Read the model definition and answer for the solid it produces. Units are mm, in the model's axes. A direction names the side the tool comes from. Round coordinates to 2 decimals unless told otherwise and drop trailing zeros. Loops run counter-clockwise (first coordinate to the right, second up) from the corner with the lowest first, then second, coordinate; pieces in that order, holes last. Notation, with made-up numbers: (34.5, 80) - (73.5, 80) arc R17 ccw to (73.5, 99) - close; hole circle Ø8 at (87.5, 49). An arc over 180 degrees is marked (long way). Use CSV: the item, a comma, the result in double quotes. Start each with the question number.
1. Given pin 1 Ø3.5 at (x, y) = (-14.5, -1.5) entering from -Z; pin 2 Ø2 at (x, z) = (-0.5, -0.5) entering from +Y; pin 3 Ø3.5 at (x, y) = (17.5, -1.5) entering from +Z, each flat-ended and moving along its own axis, determine where each tip first touches the part or whether it passes through.
2. A tool of negligible diameter and unlimited length cuts with its end or side. For faces 1 (the flat face through (0, 0, 4)), 2 (the flat face through (-8, -3, 10)), 3 (the cylindrical face through (-5.181, -2.872, 9.734)), from which of +Z, -Z, +X, -X, +Y, -Y can it reach the whole face along a straight path? Write none if from no direction.
3. Find section A-A (x = -18). Give the vertices of the cut face in (y, z) (3 decimals).
4. Determine the mould class of faces 4 (the cylindrical face through (-16.636, -3.75, 8.905)), 5 (the cylindrical face through (0.1, -2.9, 7.5)), 6 (the cylindrical face through (-23.35, -1.95, 5.06)), 7 (the flat face through (-5, -5.825, 7)) for opening direction Y: +Y half, -Y half, draft (parallel to the pull), parting line (faces both ways), or undercut.
5. Consider line 1 along Y through (x, z) = (-18, 10) (3 decimals); line 2 along Z through (x, y) = (-8.5, -0.5); line 3 along Y through (x, z) = (2, -1) (3 decimals). Determine where each line is inside the solid, lowest interval first.
6. Find section C-C (x = 18). Give the vertices of the cut face in (y, z) (3 decimals), and give its area (3 significant figures).
7. Find section D-D (x = 0). Give the vertices of the cut face in (y, z) (3 decimals).
from build123d import *

# Parameters (mm, degrees)
SKETCH3_W           = 41.4470817463862
SKETCH3_H           = 7.459999999999999
BOSS_EXTRUDE1_DEPTH = 5.825
BOSS_EXTRUDE3_DEPTH = 7.46
BOSS_EXTRUDE4_DEPTH = 5.825
SKETCH7_R           = 3.0300000000000007
CUT_EXTRUDE1_DEPTH  = 1.1
FILLET1_R           = 0.15
SKETCH8_R           = 1.8500000000000012
CUT_EXTRUDE2_DEPTH  = 26.910016764772163
FILLET2_R           = 1
FILLET3_R           = 2
SKETCH10_R          = 1.8500000000000012
BOSS_EXTRUDE5_DEPTH = 5.45
BOSS_EXTRUDE6_REACH = 30.603
SKETCH11_R          = 6
CUT_EXTRUDE3_DEPTH  = 35.90405396884001
FILLET4_R           = 1
FILLET5_R           = 2
FILLET6_R           = 4


with BuildPart() as part:
    # Sketch3 → Boss-Extrude1 (new body)
    with BuildSketch(Plane(origin=(0, 0, 0), x_dir=(1, 0, 0), z_dir=(0, 1, 0))):
        with Locations((7.11e-15, -6.269999999999988)):
            Rectangle(SKETCH3_W, SKETCH3_H)
    extrude(amount=-BOSS_EXTRUDE1_DEPTH)

    # Sketch4 → Boss-Extrude3 (add)
    with BuildSketch(Plane.XY.offset(2.5400000000000014)):
        with BuildLine():
            Line((20.72354087319311, 1e-17), (14.877501000800818, -2.18e-15))
            ThreePointArc((14.877501000800818, -2.18e-15), (17.523673872635282, 1.4715379162724416), (20.442771335934772, 0.6674703156202451))
            Line((20.442771335934772, 0.6674703156202451), (23.75850887052414, -1.8896455528490175))
            Line((23.75850887052414, -1.8896455528490175), (20.72354087319311, -5.825000000000009))
            Line((20.72354087319311, -5.825000000000009), (20.72354087319311, 1e-17))
        make_face()
        with BuildLine():
            Line((-20.723540873193116, -1.342e-14), (-20.72354087319311, -5.825000000000023))
            Line((-20.72354087319311, -5.825000000000023), (-23.75850887052414, -1.8896455528490332))
            Line((-23.75850887052414, -1.8896455528490332), (-20.442771335934772, 0.6674703156202321))
            ThreePointArc((-20.442771335934772, 0.6674703156202321), (-17.523673872635282, 1.4715379162724296), (-14.877501000800818, -1.085e-14))
            Line((-14.877501000800818, -1.085e-14), (-20.723540873193116, -1.342e-14))
        make_face()
    extrude(amount=BOSS_EXTRUDE3_DEPTH)

    # Sketch6 → Boss-Extrude4 (add)
    with BuildSketch(Plane(origin=(0, 0, 0), x_dir=(1, 0, 0), z_dir=(0, 1, 0))):
        with BuildLine():
            Line((6.000000000000012, 0), (6.000000000000012, -2.539999999999988))
            Line((6.000000000000012, -2.539999999999988), (-6.000000000000012, -2.5399999999999876))
            Line((-6.000000000000012, -2.5399999999999876), (-6.000000000000012, 0))
            ThreePointArc((-6.000000000000012, 0), (3.7e-16, 6.000000000000012), (6.000000000000012, 0))
        make_face()
    extrude(amount=-BOSS_EXTRUDE4_DEPTH)

    # Sketch7 → Cut-Extrude1 (cut)
    with BuildSketch(Plane(origin=(0, 0, 0), x_dir=(1, 0, 0), z_dir=(0, 1, 0))):
        with Locations(Location((-3.23e-15, 1.128e-14, 0), (0, 0, 270))):
            Circle(SKETCH7_R)
    extrude(amount=-CUT_EXTRUDE1_DEPTH, mode=Mode.SUBTRACT)

    # Fillet1
    fillet1_edges = [part.edges().sort_by_distance(p)[0] for p in [
        (-3.65e-15, 0, -3.030000000000012),
    ]]
    fillet(fillet1_edges, radius=FILLET1_R)

    # Sketch8 → Cut-Extrude2 (cut, through all)
    with BuildSketch(Plane(origin=(0, 0, 2.5399999999999885), x_dir=(-1, 0, 0), z_dir=(0, 0, -1))):
        with Locations((-18.000000000000007, -2.500000000000002)):
            Circle(SKETCH8_R)
        with Locations((18, -2.500000000000002)):
            Circle(SKETCH8_R)
    extrude(amount=-CUT_EXTRUDE2_DEPTH, mode=Mode.SUBTRACT)

    # Fillet2
    fillet2_edges = [part.edges().sort_by_distance(p)[0] for p in [
        (23.75850887052414, -1.8896455528490175, 6.270000000000001),
        (-23.75850887052414, -1.8896455528490332, 6.270000000000001),
    ]]
    fillet(fillet2_edges, radius=FILLET2_R)

    # Fillet3
    fillet3_edges = [part.edges().sort_by_distance(p)[0] for p in [
        (6.000000000000012, -2.9125, 2.539999999999988),
        (-6.000000000000012, -2.9125, 2.5399999999999876),
    ]]
    fillet(fillet3_edges, radius=FILLET3_R)

    # Sketch10 → Boss-Extrude5 (add)
    with BuildSketch(Plane.XY.offset(9.999999999999988)):
        with BuildLine():
            Line((-14.000000000000012, -2.500000000000014), (-14.000000000000012, -5.825000000000023))
            Line((-14.000000000000012, -5.825000000000023), (-20.72354087319311, -5.825000000000023))
            Line((-20.72354087319311, -5.825000000000023), (-23.147816036529186, -2.681513131755552))
            ThreePointArc((-23.147816036529186, -2.681513131755552), (-23.347708436606982, -1.9427104070558383), (-22.966641291612717, -1.2789527188604377))
            Line((-22.966641291612717, -1.2789527188604377), (-20.442771335934772, 0.6674703156202321))
            ThreePointArc((-20.442771335934772, 0.6674703156202321), (-16.235217484183835, 1.0896438084954059), (-14.000000000000012, -2.500000000000014))
        make_face()
        with Locations(Location((-18, -2.500000000000002, 0), (0, 0, 180))):
            Circle(SKETCH10_R, mode=Mode.SUBTRACT)
    extrude(amount=BOSS_EXTRUDE5_DEPTH)

    # Boss-Extrude6: up to this face of the body (flat: up to its plane)
    boss_extrude6_end = Plane(part.part.faces().sort_by_distance((-1.463911486, -5.825, 5.299880687))[0])
    # Sketch9 → Boss-Extrude6 (add, up to the picked face)
    with BuildSketch(Plane(origin=(0, 0, 0), x_dir=(1, 0, 0), z_dir=(0, 1, 0)), mode=Mode.PRIVATE) as boss_extrude6_sk1:
        with BuildLine():
            Line((-20.723540873193105, -8.650000000000004), (-28.322297461263148, -8.650000000000004))
            ThreePointArc((-28.322297461263148, -8.650000000000004), (-29.466272655610958, -8.848231620695078), (-30.476852522423187, -9.41981132075475))
            ThreePointArc((-30.476852522423187, -9.41981132075475), (-30.58177170288316, -10.475269498785284), (-29.5263135248526, -10.580188679245284))
            ThreePointArc((-29.5263135248526, -10.580188679245284), (-26.4222974612631, -12.050000000000004), (-29.5263135248526, -13.519811320754725))
            ThreePointArc((-29.5263135248526, -13.519811320754725), (-30.581771702883188, -13.624730501214703), (-30.476852522423194, -14.680188679245271))
            ThreePointArc((-30.476852522423194, -14.680188679245271), (-29.466272655610975, -15.251768379304975), (-28.322297461263148, -15.450000000000019))
            Line((-28.322297461263148, -15.450000000000019), (-20.723540873193105, -15.450000000000003))
            Line((-20.723540873193105, -15.450000000000003), (-20.723540873193105, -8.650000000000004))
        make_face()
    boss_extrude6_tool1 = split(extrude(boss_extrude6_sk1.sketch, amount=-BOSS_EXTRUDE6_REACH, mode=Mode.PRIVATE), bisect_by=boss_extrude6_end, keep=Keep.BOTH, mode=Mode.PRIVATE)
    add(boss_extrude6_tool1.solids().sort_by(Axis((-24.875622, 0, 12.05), (0, -1, 0)))[0])

    # Sketch11 → Cut-Extrude3 (cut, through all)
    with BuildSketch(Plane(origin=(0, 0, 0), x_dir=(1, 0, 0), z_dir=(0, 1, 0))):
        with Locations((1.06e-15, -13.500000000000007)):
            Circle(SKETCH11_R)
    extrude(amount=-CUT_EXTRUDE3_DEPTH, mode=Mode.SUBTRACT)

    # Fillet4
    fillet4_edges = [part.edges().sort_by_distance(p)[0] for p in [
        (-23.34770843660698, -1.9427104070558383, 8.650000000000004),
        (-22.137450955112786, -0.6394763594302192, 8.650000000000004),
        (-21.935678454861147, -4.253256565877788, 8.650000000000006),
    ]]
    fillet(fillet4_edges, radius=FILLET4_R)

    # Fillet5
    fillet5_edges = [part.edges().sort_by_distance(p)[0] for p in [
        (-21.30826061861286, -1.1e-16, 11.55),
    ]]
    fillet(fillet5_edges, radius=FILLET5_R)

    # Fillet6
    fillet6_edges = [part.edges().sort_by_distance(p)[0] for p in [
        (-14.225745371812032, -1.1752351145952094, 9.999999999999988),
        (-14.000000000000012, -4.162500000000019, 9.999999999999988),
        (4.873397172404469, -2.9125, 9.999999999999988),
        (-4.873397172404467, -2.9125, 9.999999999999988),
    ]]
    fillet(fillet6_edges, radius=FILLET6_R)


solid = part.part
Filled sheet:
1,pin 1,"stops at z = 2.54"
1,pin 2,"stops at y = -1.1"
1,pin 3,"stops at z = 10"
2,face 1,"+Z, -Z, +Y"
2,face 2,"+Z, +X, +Y, -Y"
2,face 3,"+Z, +Y, -Y"
3,outline,"(-5.825, 2.54) - (-4.35, 2.54) - (-4.35, 15.45) - (-5.825, 15.45) - close; (-0.65, 2.54) - (1.5, 2.54) - (1.5, 15.45) - (-0.65, 15.45) - close"
4,face 4,"undercut"
4,face 5,"draft"
4,face 6,"parting line"
4,face 7,"-Y half"
5,line 1,"y = -5.825 to -4.35, -0.65 to 1.5"
5,line 2,"z = 2.54 to 10"
5,line 3,"y = -5.825 to -1.1"
6,outline,"(-5.825, 2.54) - (-4.35, 2.54) - (-4.35, 10) - (-5.825, 10) - close; (-0.65, 2.54) - (1.5, 2.54) - (1.5, 10) - (-0.65, 10) - close"
6,area,"27.0 mm²"
7,outline,"(-5.825, -6) - (0, -6) - (0, -3.18) arc R0.15 ccw to (-0.15, -3.03) - (-1.1, -3.03) - (-1.1, 3.03) - (-0.15, 3.03) arc R0.15 ccw to (0, 3.18) - (0, 7.5) - (-5.825, 7.5) - close"
